Check sheet for the modelled part. Datum: model origin and axes. Units: mm. Face numbers are marked on the shaded views. A direction names the side the tool comes from. Coordinates: 2 decimals unless noted, no trailing zeros. Loops run counter-clockwise (first coordinate to the right, second up) from the corner with the lowest first, then second, coordinate; pieces in that order, holes last. Notation, with made-up numbers: M 20,70.25 L 78,70.25 A18 cw 78,82.25 Z; hole C 27.25,82 d9. An arc over 180 degrees is marked long. Answer as CSV lines item,"result". Start each with the question number.
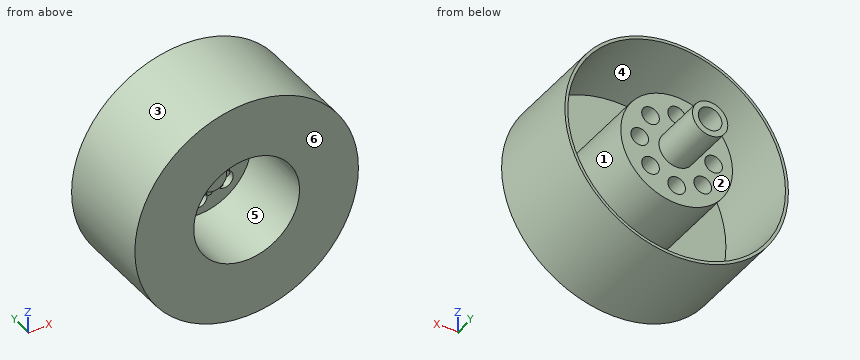
from build123d import *

# Parameters (mm, degrees)
F0_R      = 19
F1_DEPTH  = 17
F2_R      = 9
F3_DEPTH  = 13
F4_R      = 1.5
F5_DEPTH  = 25
F6_R      = 4.25
F7_DEPTH  = 2
F8_R      = 2.25
F9_DEPTH  = 2.1
F10_R     = 0.5
F11_DEPTH = 1
F12_R     = 3
F12_R_2   = 2
F13_DEPTH = 9
F15_R     = 18.5
F15_R_2   = 9.5
F16_DEPTH = 16


with BuildPart() as f1:
    # F0 (on Front) → F1 (new body)
    with BuildSketch(Plane.XZ):
        Circle(F0_R)
    extrude(amount=-F1_DEPTH)

    # F2 (on face) → F3 (cut)
    with BuildSketch(Plane.XZ):
        Circle(F2_R)
    extrude(amount=-F3_DEPTH, mode=Mode.SUBTRACT)

    # F4 (on face) → F5 (cut)
    with BuildSketch(Plane.XZ.offset(-13)):
        with Locations((0, 6.275373)):
            Circle(F4_R)
        with Locations((4.437359, 4.437359)):
            Circle(F4_R)
        with Locations((6.275373, 0)):
            Circle(F4_R)
        with Locations((4.437359, -4.437359)):
            Circle(F4_R)
        with Locations((0, -6.275373)):
            Circle(F4_R)
        with Locations((-4.437359, -4.437359)):
            Circle(F4_R)
        with Locations((-6.275373, 0)):
            Circle(F4_R)
        with Locations((-4.437359, 4.437359)):
            Circle(F4_R)
    extrude(amount=-F5_DEPTH, mode=Mode.SUBTRACT)

    # F6 (on face) → F7 (join)
    with BuildSketch(Plane.XZ.offset(-13)):
        Circle(F6_R)
    extrude(amount=F7_DEPTH)

    # F8 (on face) → F9 (join)
    with BuildSketch(Plane.XZ.offset(-11)):
        Circle(F8_R)
    extrude(amount=F9_DEPTH)

    # F10 (on face) → F11 (join)
    with BuildSketch(Plane.XZ.offset(-11)):
        with Locations((0, 3.12862)):
            Circle(F10_R)
        with Locations((1.838957, 2.531107)):
            Circle(F10_R)
        with Locations((2.975495, 0.966797)):
            Circle(F10_R)
        with Locations((2.975495, -0.966797)):
            Circle(F10_R)
        with Locations((1.838957, -2.531107)):
            Circle(F10_R)
        with Locations((0, -3.12862)):
            Circle(F10_R)
        with Locations((-1.838957, -2.531107)):
            Circle(F10_R)
        with Locations((-2.975495, -0.966797)):
            Circle(F10_R)
        with Locations((-2.975495, 0.966797)):
            Circle(F10_R)
        with Locations((-1.838957, 2.531107)):
            Circle(F10_R)
    extrude(amount=F11_DEPTH)

    # F12 (on face) → F13 (join)
    with BuildSketch(Plane(origin=(0, 17, 0), x_dir=(-1, 0, 0), z_dir=(0, 1, 0))):
        Circle(F12_R)
        Circle(F12_R_2, mode=Mode.SUBTRACT)
    extrude(amount=F13_DEPTH)

    # F15 (on face) → F16 (cut)
    with BuildSketch(Plane(origin=(0, 17, 0), x_dir=(-1, 0, 0), z_dir=(0, 1, 0))):
        Circle(F15_R)
        Circle(F15_R_2, mode=Mode.SUBTRACT)
    extrude(amount=-F16_DEPTH, mode=Mode.SUBTRACT)


solid = f1.part
Item 1: Sectioned sample at A-A, the plane y = 14.75. Give the number of separate pieces and of enclosed holes in the cut face, and give its area (3 significant figures).
Item 2: Go/stop test with flat-tipped pins: pin 1 (5 mm diameter, centred on x = -4.44, z = 4.44, fed in from +Y); pin 2 (0.8 mm diameter, centred on x = -3, z = -1, fed in from -Y); pin 3 (4 mm diameter, centred on x = -6.28, z = 0, fed in from -Y). Record where each tip stops, or that it passes through.
Item 3: Sectioned sample at B-B, the plane x = -6.5. Record the boundary of the cut face in (y, z), and give its area (3 significant figures).
Item 4: Set-up check for the marked faces 4, 5 and 6: record each of +Z, -Z, +X, -X, +Y, -Y from which the full face is reachable in a straight line by a thin tool's end or side.
Item 5: Sectioned sample at D-D, the plane x = 8.5. Record the boundary of the cut face in (y, z), and give its area (3 significant figures).
Item 6: Material ranges on line 1 (Z direction, x = 0, y = 11.25); line 2 (X direction, y = 16, z = -4); line 3 (Z direction, x = -5, y = 5.5), recorded low to high. Write a range as from..to.
Item 7: Release check for a two-part mould opening along X. For the marked faces 1, 2 and 3 record: released by +X, released by -X, zero draft, split by the parting line, or undercut.
Item 8: Sectioned sample at C-C, the plane y = 22.25. Record the boundary of the cut face in (x, z), and give its area (3 significant figures).
Reply:
1,separate pieces,"2"
1,enclosed holes,"9"
1,area,"286 mm²"
2,pin 1,"y = 17"
2,pin 2,"y = 10"
2,pin 3,"y = 13"
3,outline,"M 0,-17.85 L 17,-17.85 L 17,-17.32 L 1,-17.32 L 1,-6.93 L 17,-6.93 L 17,-1.48 L 13,-1.48 L 13,-6.22 L 0,-6.22 Z; M 0,6.22 L 13,6.22 L 13,1.48 L 17,1.48 L 17,6.93 L 1,6.93 L 1,17.32 L 17,17.32 L 17,17.85 L 0,17.85 Z"
3,area,"101 mm²"
4,face 4,"+Y"
4,face 5,"-Y"
4,face 6,"+Z, -Z, +X, -X, -Y"
5,outline,"M 0,-16.99 L 17,-16.99 L 17,-16.43 L 1,-16.43 L 1,-4.24 L 17,-4.24 L 17,4.24 L 1,4.24 L 1,16.43 L 17,16.43 L 17,16.99 L 0,16.99 L 0,2.96 L 13,2.96 L 13,-2.96 L 0,-2.96 Z"
5,area,"111 mm²"
6,line 1,"-19..-18.5, -9.5..-9, -4.25..4.25, 9..9.5, 18.5..19"
6,line 2,"-18.57..-18.06, -8.62..-5.87, -3..3, 5.87..8.62, 18.06..18.57"
6,line 3,"-18.33..-17.81, -8.08..-7.48, 7.48..8.08, 17.81..18.33"
7,face 1,"undercut"
7,face 2,"zero draft"
7,face 3,"split by the parting line"
8,outline,"C 0,0 d6; hole C 0,0 d4"
8,area,"15.7 mm²"
